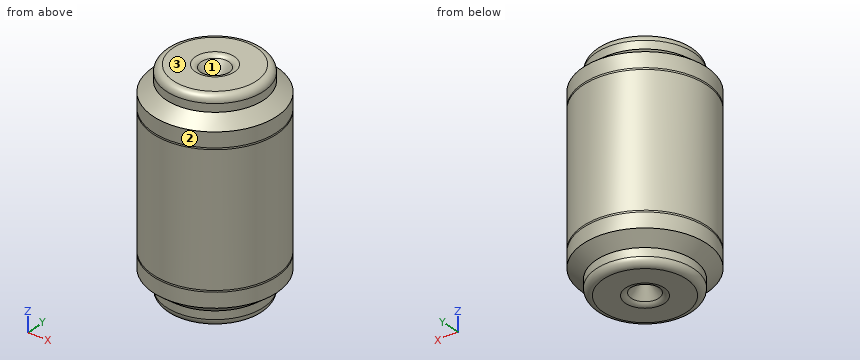
from build123d import *

# Parameters (mm, degrees)
F2_R = 5.08


with BuildPart() as f1:
    # F0 (on Front) → F1 (revolve)
    with BuildSketch(Plane.XZ):
        with BuildLine():
            Line((0, -61.158732), (0, 62.042959))
            Line((0, 62.042959), (-11.49489, 76.779999))
            Line((-11.49489, 76.779999), (-35.07416, 76.779999))
            Line((-35.07416, 76.779999), (-35.07416, 65.874591))
            Line((-35.07416, 65.874591), (-44.505868, 58.506068))
            Line((-44.505868, 58.506068), (-44.505868, -46.716429))
            ThreePointArc((-44.505868, -46.716429), (-40.659053, -56.89148), (-30.653045, -61.158732))
            Line((-30.653045, -61.158732), (0, -61.158732))
        make_face()
    revolve(axis=Axis((0, 0, 0.442114), (0, 0, -1)))

    # F2
    f2_edges = [f1.edges().sort_by_distance(p)[0] for p in [
        (11.49489, 0, 76.779999),
        (35.07416, 0, 76.779999),
    ]]
    fillet(f2_edges, radius=F2_R)

    # F3: F1 across plane


with BuildPart() as f1_1:
    add(f1.part)
    add(f1.part.mirror(Plane.XY))


solid = f1_1.part
Part model, mm, in its own coordinate system. Face numbers are marked on the shaded views. Coordinates: 2 decimals unless noted, no trailing zeros. Order: outer loops, then holes, each group sorted by start corner. A loop starts at its lowest first (then second) coordinate and runs counter-clockwise, first axis right, second up.
(1) Probe L1, parallel to X at y = -3, z = -67; L2, parallel to X at y = 1, z = 39; L3, parallel to Y at x = -8.5, z = 7.5. List the from-to ranges inside material, lowest first.
Check sheet entries:
L1: x = -34.95 to -2.44, 2.44 to 34.95
L2: x = -44.49 to 44.49
L3: y = -43.69 to 43.69
(2) Pin check, flat tips, straight feed: pin 1 Ø10 at (y, z) = (14.5, 44.5) entering from +X; pin 2 Ø10 at (x, z) = (-30, 13.5) entering from -Y; pin 3 Ø6 at (y, z) = (-10, -37) entering from -X. Stop position of each tip, or through.
Check sheet entries:
pin 1: stops at x = 43.48
pin 2: stops at y = -36.82
pin 3: stops at x = -43.95
(3) Pull direction X, two halves, no side cores. Call the marked faces 1, 2 and 3: pulls with the +X half, pulls with the -X half, needs draft (parallel to the pull), parting line crosses it, or undercut.
Check sheet entries:
face 1: undercut
face 2: parting line crosses it
face 3: needs draft
(4) Slice it at A-A, the plane z = 21. Write the cut outline in (x, y), and give its area (3 significant figures).
Check sheet entries:
outline: circle Ø89.01 at (0, 0)
area: 6,220 mm2
